```python
from build123d import *

# Parameters (mm, degrees)
BOSS_EXTRU_1_DEPTH      = 5.5
ESQUISSE2_R             = 12.5
ESQUISSE2_R_2           = 5
BOSS_EXTRU_2_DEPTH      = 10
ENL_V_START             = -10
ESQUISSE3_R             = 5
ENL_V_MAT_EXTRU_1_DEPTH = 10
ESQUISSE4_R             = 3.5
ENL_V_MAT_EXTRU_2_DEPTH = 10
D_GAGEMENT_M61_D        = 7
D_GAGEMENT_M61_DEPTH    = 120
D_GAGEMENT_M61_TIP      = 2.103012167
D_GAGEMENT_M62_D        = 7
D_GAGEMENT_M62_DEPTH    = 120
D_GAGEMENT_M62_TIP      = 2.103012167


with BuildPart() as part:
    # Esquisse1 → Boss.-Extru.1 (new body)
    with BuildSketch(Plane(origin=(0, 0, 0), x_dir=(1, 0, 0), z_dir=(0, 1, 0))):
        with BuildLine():
            Line((-9.949874371, 15), (-5, 30))
            Line((-5, 30), (5, 30))
            Line((5, 30), (9.949874371, 15))
            ThreePointArc((9.949874371, 15), (18, 0), (9.949874371, -15))
            Line((9.949874371, -15), (5, -30))
            Line((5, -30), (-5, -30))
            Line((-5, -30), (-9.949874371, -15))
            ThreePointArc((-9.949874371, -15), (-18, 0), (-9.949874371, 15))
        make_face()
    extrude(amount=BOSS_EXTRU_1_DEPTH)

    # Esquisse2 → Boss.-Extru.2 (add)
    with BuildSketch(Plane(origin=(0, 5.5, 0), x_dir=(1, 0, 0), z_dir=(0, 1, 0))):
        with Locations(Location((0, 0, 0), (0, 0, 90))):
            Circle(ESQUISSE2_R)
        with Locations(Location((0, 0, 0), (0, 0, 270))):
            Circle(ESQUISSE2_R_2, mode=Mode.SUBTRACT)
    extrude(amount=BOSS_EXTRU_2_DEPTH)

    # Esquisse3 → Enlèv. mat.-Extru.1 (cut)
    with BuildSketch(Plane(origin=(0, 5.5, 0), x_dir=(1, 0, 0), z_dir=(0, 1, 0)).offset(ENL_V_START)):
        with Locations(Location((0, 0, 0), (0, 0, 90))):
            Circle(ESQUISSE3_R)
    extrude(amount=ENL_V_MAT_EXTRU_1_DEPTH, mode=Mode.SUBTRACT)

    # Esquisse4 → Enlèv. mat.-Extru.2 (cut)
    with BuildSketch(Plane(origin=(0, 5.5, 0), x_dir=(1, 0, 0), z_dir=(0, 1, 0))):
        with Locations(Location((0, 22.5, 0), (0, 0, 270))):
            Circle(ESQUISSE4_R)
        with Locations(Location((0, -22.5, 0), (0, 0, 270))):
            Circle(ESQUISSE4_R)
    extrude(amount=-ENL_V_MAT_EXTRU_2_DEPTH, mode=Mode.SUBTRACT)

    # Dégagement M61
    with Locations(Plane(origin=(0, 0, 0), x_dir=(0, 0, -1), z_dir=(0, 1, 0))):
        with Locations((22.5, 0), (-22.5, 0)):
            Hole(D_GAGEMENT_M61_D / 2, depth=D_GAGEMENT_M61_DEPTH)
            with Locations((0, 0, -(D_GAGEMENT_M61_DEPTH + D_GAGEMENT_M61_TIP / 2))):  # 118° drill point
                Cone(0, D_GAGEMENT_M61_D / 2, D_GAGEMENT_M61_TIP, mode=Mode.SUBTRACT)

    # Dégagement M62
    with Locations(Plane(origin=(0, -60, 0), x_dir=(0, 0, 1), z_dir=(0, -1, 0))):
        with Locations((22.5, 0), (-22.5, 0)):
            Hole(D_GAGEMENT_M62_D / 2, depth=D_GAGEMENT_M62_DEPTH)
            with Locations((0, 0, -(D_GAGEMENT_M62_DEPTH + D_GAGEMENT_M62_TIP / 2))):  # 118° drill point
                Cone(0, D_GAGEMENT_M62_D / 2, D_GAGEMENT_M62_TIP, mode=Mode.SUBTRACT)


solid = part.part
```
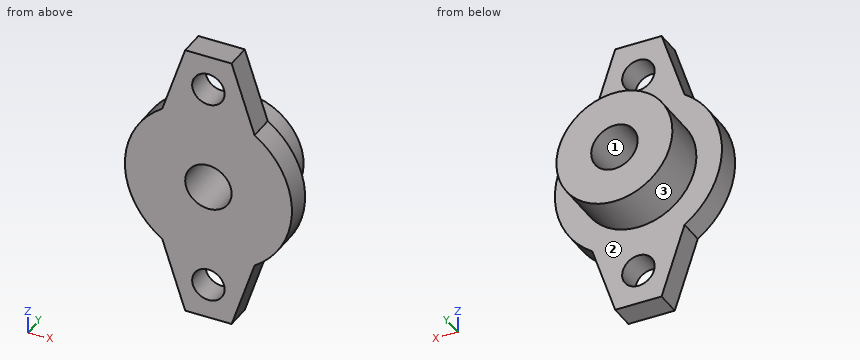
Work out the finished part from the listing and answer in its coordinate system (mm). Face numbers are marked on the shaded views. Give positions to 0.01 mm unless a question says otherwise; leave off trailing zeros. Loops run counter-clockwise (first coordinate to the right, second up) from the corner with the lowest first, then second, coordinate; pieces in that order, holes last. Notation, with made-up numbers: M 43.5,2.5 L 90.5,2.5 A13 cw 90.5,9.5 Z; hole C 64,81.5 d2. An arc over 180 degrees is marked long. One line per item, written item: value. Start each with the question number.
1. Find section C-C (y = 3.25). Give the vertices of the cut face in (x, z), and give its area (3 significant figures).
2. Each of these flat-tipped pins is pushed along its axis until it touches: P1, Ø4, axis at x = 7.5, z = 14.5, coming from the +Y side; P2, Ø1, axis at y = 1.5, z = -8.5, coming from the -X side; P3, Ø1, axis at x = 13.5, y = 3, coming from the -Z side. Where does it stop, or does it pass through?
3. Find section B-B (x = 0). Give the vertices of the cut face in (y, z).
4. Find section A-A (z = 0). Give the vertices of the cut face in (x, y), and give its area (3 significant figures).
5. Determine the mould class of the marked faces 1, 2 and 3 for opening direction X: released by +X, released by -X, zero draft, split by the parting line, or undercut.
6. Find section D-D (y = 14). Give the vertices of the cut face in (x, z).
7. Find the intervals of material crossed by probe 1 along X at (y, z) = (7, 0); probe 2 along Y at (x, z) = (-14.5, -2.5); probe 3 along X at (y, z) = (4, 0), in increasing order.
Reported:
1. outline: M -9.95,-15 L -5,-30 L 5,-30 L 9.95,-15 A18 ccw 9.95,15 L 5,30 L -5,30 L -9.95,15 A18 ccw Z; hole C 0,0 d10; hole C 0,-22.5 d7; hole C 0,22.5 d7
1. area: 1,230 mm²
2. P1: stops at y = 5.5
2. P2: stops at x = -16.12
2. P3: stops at z = -12.45
3. outline: M 0,-30 L 5.5,-30 L 5.5,-26 L 0,-26 Z; M 0,-19 L 5.5,-19 L 5.5,-12.5 L 15.5,-12.5 L 15.5,-5 L 0,-5 Z; M 0,5 L 15.5,5 L 15.5,12.5 L 5.5,12.5 L 5.5,19 L 0,19 Z; M 0,26 L 5.5,26 L 5.5,30 L 0,30 Z
4. outline: M -18,0 L -5,0 L -5,15.5 L -12.5,15.5 L -12.5,5.5 L -18,5.5 Z; M 5,0 L 18,0 L 18,5.5 L 12.5,5.5 L 12.5,15.5 L 5,15.5 Z
4. area: 293 mm²
5. face 1: undercut
5. face 2: zero draft
5. face 3: split by the parting line
6. outline: C 0,0 d25; hole C 0,0 d10
7. probe 1: x = -12.5 to -5, 5 to 12.5
7. probe 2: y = 0 to 5.5
7. probe 3: x = -18 to -5, 5 to 18
